Verification items for the finished model (mm, model axes). Give positions to 0.01 mm unless a question says otherwise; leave off trailing zeros. Write each loop counter-clockwise with the first axis right and the second up, starting at its lowest first coordinate (ties: lowest second). Pieces come first, ordered by that corner, then holes. Notation, with made-up numbers: (15.25, 45.25) -> (63.25, 45.25) arc R3 ccw to (63.25, 50.25) -> close; hole circle Ø5 at (-35.5, 76). An arc over 180 degrees is marked (long way). Use one line per item in the form item = value. Start each with the question number.
(1) Section check B-B, the plane x = -6. Record the cut outline in (y, z).
(2) Scan lines: L1, parallel to X at y = 1.15, z = -35.5; L2, parallel to Z at x = -11.25, y = 0.7; L3, parallel to X at y = 1.3, z = 34.5. Record each from-to range of solid material in increasing order.
(3) Release check for a two-part mould opening along Z. For faces 1 (the face through (-1, 1, -38.1)), 2 (the face through (2.51, 1.48, 27.44)), 3 (the face through (13.019, 1, 0)) record: pulls with the +Z half, pulls with the -Z half, needs draft (parallel to the pull), parting line crosses it, or undercut.
(4) Section check C-C, the plane y = 1.45. Record the cut outline in (x, z).
(5) Section check A-A, the plane z = 17.9. Record the cut outline in (x, y), plus the area to 3 significant figures.
(6) Depth check by flat-ended pin: pin 1 Ø2.5 at (x, z) = (10.39, 35.5) entering from -Y. Enter the tip coordinate at first touch or a pass-through.
from build123d import *

# Parameters (mm, degrees)
SKETCH1_R           = 1.1
SKETCH1_R_2         = 10
BOSS_EXTRUDE1_DEPTH = 3


with BuildPart() as part:
    # Sketch1 → Boss-Extrude1 (new body)
    with BuildSketch(Plane(origin=(0, 0, 0), x_dir=(1, 0, 0), z_dir=(0, 1, 0))):
        with BuildLine():
            Line((-13.01875, -38.1), (10.51875, -38.1))
            ThreePointArc((10.51875, -38.1), (12.286516953, -37.367766953), (13.01875, -35.6))
            Line((13.01875, -35.6), (13.01875, 35.6))
            ThreePointArc((13.01875, 35.6), (12.286516953, 37.367766953), (10.51875, 38.1))
            Line((10.51875, 38.1), (-13.01875, 38.1))
            Line((-13.01875, 38.1), (-13.01875, -38.1))
        make_face()
        with Locations(Location((-11.38125, 35.5, 0), (0, 0, 270))):
            Circle(SKETCH1_R, mode=Mode.SUBTRACT)
        with Locations(Location((10.39375, 35.5, 0), (0, 0, 270))):
            Circle(SKETCH1_R, mode=Mode.SUBTRACT)
        with Locations(Location((-11.38125, -35.5, 0), (0, 0, 270))):
            Circle(SKETCH1_R, mode=Mode.SUBTRACT)
        with Locations(Location((10.39375, -35.5, 0), (0, 0, 270))):
            Circle(SKETCH1_R, mode=Mode.SUBTRACT)
        with Locations(Location((-0.49375, -17.9, 0), (0, 0, 270))):
            Circle(SKETCH1_R_2, mode=Mode.SUBTRACT)
    extrude(amount=BOSS_EXTRUDE1_DEPTH)


solid = part.part
Completed:
q1.outline = (0, -38.1) -> (3, -38.1) -> (3, 9.55) -> (0, 9.55) -> close; (0, 26.25) -> (3, 26.25) -> (3, 38.1) -> (0, 38.1) -> close
q2.L1 = -13.02 to -12.48, -10.28 to 9.29, 11.49 to 13.02
q2.L2 = -38.1 to -36.59, -34.41 to 34.41, 36.59 to 38.1
q2.L3 = -13.02 to -11.84, -10.92 to 9.94, 10.85 to 13.02
q3.face_1 = pulls with the -Z half
q3.face_2 = undercut
q3.face_3 = needs draft
q4.outline = (-13.02, -38.1) -> (10.52, -38.1) arc R2.5 ccw to (13.02, -35.6) -> (13.02, 35.6) arc R2.5 ccw to (10.52, 38.1) -> (-13.02, 38.1) -> close; hole circle Ø2.2 at (-11.38, -35.5); hole circle Ø2.2 at (-11.38, 35.5); hole circle Ø20 at (-0.49, 17.9); hole circle Ø2.2 at (10.39, -35.5); hole circle Ø2.2 at (10.39, 35.5)
q5.outline = (-13.02, 0) -> (-10.49, 0) -> (-10.49, 3) -> (-13.02, 3) -> close; (9.51, 0) -> (13.02, 0) -> (13.02, 3) -> (9.51, 3) -> close
q5.area = 18.1 mm²
q6.pin_1 = 0
